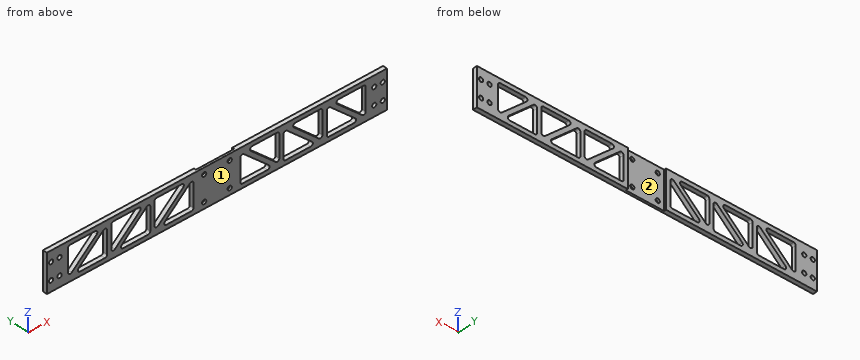
```python
from build123d import *

# Parameters (mm, degrees)
SKETCH2_W                   = 57.15
SKETCH2_H                   = 6.35
BOSS_EXTRUDE2_DEPTH         = 254
F_1_4_0_25_DIAMETER_HOLE1_D = 6.35
CUT_EXTRUDE1_REACH          = 257.681
FILLET1_R                   = 3.175
FILLET1_OF_MIRROR4_R        = 3.175
SKETCH7_W                   = 57.15
SKETCH7_H                   = 57.15
CUT_EXTRUDE2_DEPTH          = 3.175
F_1_4_0_25_DIAMETER_HOLE2_D = 6.35


with BuildPart() as part:
    # Sketch2 → Boss-Extrude2 (new, symmetric)
    with BuildSketch(Plane(origin=(0, 0, 0), x_dir=(0, 0, -1), z_dir=(1, 0, 0))):
        Rectangle(SKETCH2_W, SKETCH2_H)
    extrude(amount=BOSS_EXTRUDE2_DEPTH, both=True)

    # 1/4 (0.25) Diameter Hole1 (through all)
    with Locations(Plane(origin=(0, 3.175, 0), x_dir=(1, 0, 0), z_dir=(0, 1, 0))):
        with Locations((-247.65, -12.7), (-247.65, 12.7), (-234.95, 12.7), (-234.95, -12.7)):
            f_1_4_0_25_diameter_hole1 = Hole(F_1_4_0_25_DIAMETER_HOLE1_D / 2)

    # Mirror1: 1/4 (0.25) Diameter Hole1 across plane
    add(f_1_4_0_25_diameter_hole1.mirror(Plane(origin=(0, 0, 0), x_dir=(0, 0, 1), z_dir=(1, 0, 0))), mode=Mode.SUBTRACT)

    # Sketch6 → Cut-Extrude1 (cut, up to next)
    with BuildSketch(Plane(origin=(0, 3.175, 0), x_dir=(1, 0, 0), z_dir=(0, 1, 0)), mode=Mode.PRIVATE) as cut_extrude1_sk1:
        Polygon((-222.25, 22.225), (-222.25, -22.225), (-173.469521198, -22.225), align=None)
    cut_extrude1_tool1 = extrude(cut_extrude1_sk1.sketch, amount=-CUT_EXTRUDE1_REACH, mode=Mode.PRIVATE) & part.part
    # Sketch6 → Cut-Extrude1 (cut, up to next)
    with BuildSketch(Plane(origin=(0, 3.175, 0), x_dir=(1, 0, 0), z_dir=(0, 1, 0)), mode=Mode.PRIVATE) as cut_extrude1_sk2:
        Polygon((-212.822145469, 22.225), (-164.041666667, -22.225), (-164.041666667, 22.225), align=None)
    cut_extrude1_tool2 = extrude(cut_extrude1_sk2.sketch, amount=-CUT_EXTRUDE1_REACH, mode=Mode.PRIVATE) & part.part
    # Sketch6 → Cut-Extrude1 (cut, up to next)
    with BuildSketch(Plane(origin=(0, 3.175, 0), x_dir=(1, 0, 0), z_dir=(0, 1, 0)), mode=Mode.PRIVATE) as cut_extrude1_sk3:
        Polygon((-157.691666667, 22.225), (-157.691666667, -22.225), (-108.911187865, -22.225), align=None)
    cut_extrude1_tool3 = extrude(cut_extrude1_sk3.sketch, amount=-CUT_EXTRUDE1_REACH, mode=Mode.PRIVATE) & part.part
    # Sketch6 → Cut-Extrude1 (cut, up to next)
    with BuildSketch(Plane(origin=(0, 3.175, 0), x_dir=(1, 0, 0), z_dir=(0, 1, 0)), mode=Mode.PRIVATE) as cut_extrude1_sk4:
        Polygon((-148.263812135, 22.225), (-99.483333333, -22.225), (-99.483333333, 22.225), align=None)
    cut_extrude1_tool4 = extrude(cut_extrude1_sk4.sketch, amount=-CUT_EXTRUDE1_REACH, mode=Mode.PRIVATE) & part.part
    # Sketch6 → Cut-Extrude1 (cut, up to next)
    with BuildSketch(Plane(origin=(0, 3.175, 0), x_dir=(1, 0, 0), z_dir=(0, 1, 0)), mode=Mode.PRIVATE) as cut_extrude1_sk5:
        Polygon((-93.133333333, 22.225), (-93.133333333, -22.225), (-44.352854531, -22.225), align=None)
    cut_extrude1_tool5 = extrude(cut_extrude1_sk5.sketch, amount=-CUT_EXTRUDE1_REACH, mode=Mode.PRIVATE) & part.part
    # Sketch6 → Cut-Extrude1 (cut, up to next)
    with BuildSketch(Plane(origin=(0, 3.175, 0), x_dir=(1, 0, 0), z_dir=(0, 1, 0)), mode=Mode.PRIVATE) as cut_extrude1_sk6:
        Polygon((-83.705478802, 22.225), (-34.925, -22.225), (-34.925, 22.225), align=None)
    cut_extrude1_tool6 = extrude(cut_extrude1_sk6.sketch, amount=-CUT_EXTRUDE1_REACH, mode=Mode.PRIVATE) & part.part
    cut_extrude1_1 = cut_extrude1_tool1.solids().sort_by_distance((-205.98984, 3.175, 7.408333))[0]
    add(cut_extrude1_1, mode=Mode.SUBTRACT)
    cut_extrude1_2 = cut_extrude1_tool2.solids().sort_by_distance((-180.301826, 3.175, -7.408333))[0]
    add(cut_extrude1_2, mode=Mode.SUBTRACT)
    cut_extrude1_3 = cut_extrude1_tool3.solids().sort_by_distance((-141.431507, 3.175, 7.408333))[0]
    add(cut_extrude1_3, mode=Mode.SUBTRACT)
    cut_extrude1_4 = cut_extrude1_tool4.solids().sort_by_distance((-115.743493, 3.175, -7.408333))[0]
    add(cut_extrude1_4, mode=Mode.SUBTRACT)
    cut_extrude1_5 = cut_extrude1_tool5.solids().sort_by_distance((-76.873174, 3.175, 7.408333))[0]
    add(cut_extrude1_5, mode=Mode.SUBTRACT)
    cut_extrude1_6 = cut_extrude1_tool6.solids().sort_by_distance((-51.18516, 3.175, -7.408333))[0]
    add(cut_extrude1_6, mode=Mode.SUBTRACT)
    cut_extrude1 = cut_extrude1_1 + cut_extrude1_2 + cut_extrude1_3 + cut_extrude1_4 + cut_extrude1_5 + cut_extrude1_6  # Cut-Extrude1 as one shape, for the pattern or mirror that repeats it

    # Fillet1
    fillet1_edges = [part.edges().sort_by_distance(p)[0] for p in [
        (-93.133333333, 0, -22.225),
        (-44.352854531, 0, 22.225),
        (-93.133333333, 0, 22.225),
        (-83.705478802, 0, -22.225),
        (-34.925, 0, -22.225),
        (-34.925, 0, 22.225),
        (-222.25, 0, -22.225),
        (-173.469521198, 0, 22.225),
        (-222.25, 0, 22.225),
        (-212.822145469, 0, -22.225),
        (-164.041666667, 0, -22.225),
        (-164.041666667, 0, 22.225),
        (-157.691666667, 0, -22.225),
        (-108.911187865, 0, 22.225),
        (-157.691666667, 0, 22.225),
        (-148.263812135, 0, -22.225),
        (-99.483333333, 0, -22.225),
        (-99.483333333, 0, 22.225),
    ]]
    fillet(fillet1_edges, radius=FILLET1_R)

    # Mirror4: Cut-Extrude1 across plane
    add(cut_extrude1.mirror(Plane(origin=(0, 0, 0), x_dir=(0, 0, 1), z_dir=(1, 0, 0))), mode=Mode.SUBTRACT)

    # Fillet1 of Mirror4
    fillet1_of_mirror4_edges = [part.edges().sort_by_distance(p)[0] for p in [
        (93.133333333, 0, -22.225),
        (44.352854531, 0, 22.225),
        (93.133333333, 0, 22.225),
        (83.705478802, 0, -22.225),
        (34.925, 0, -22.225),
        (34.925, 0, 22.225),
        (222.25, 0, -22.225),
        (173.469521198, 0, 22.225),
        (222.25, 0, 22.225),
        (212.822145469, 0, -22.225),
        (164.041666667, 0, -22.225),
        (164.041666667, 0, 22.225),
        (157.691666667, 0, -22.225),
        (108.911187865, 0, 22.225),
        (157.691666667, 0, 22.225),
        (148.263812135, 0, -22.225),
        (99.483333333, 0, -22.225),
        (99.483333333, 0, 22.225),
    ]]
    fillet(fillet1_of_mirror4_edges, radius=FILLET1_OF_MIRROR4_R)

    # Sketch7 → Cut-Extrude2 (cut)
    with BuildSketch(Plane(origin=(0, 3.175, 0), x_dir=(1, 0, 0), z_dir=(0, 1, 0))):
        Rectangle(SKETCH7_W, SKETCH7_H)
    extrude(amount=-CUT_EXTRUDE2_DEPTH, mode=Mode.SUBTRACT)

    # 1/4 (0.25) Diameter Hole2 (through all)
    with Locations(Plane(origin=(0, 0, 0), x_dir=(1, 0, 0), z_dir=(0, 1, 0))):
        with Locations((19.05, -19.05), (-19.05, 19.05), (-19.05, -19.05), (19.05, 19.05)):
            Hole(F_1_4_0_25_DIAMETER_HOLE2_D / 2)


solid = part.part
```
Geometry: final body of the model. Coordinates: model frame, mm. Face numbers are marked on the shaded views. Round coordinates to 2 decimals unless told otherwise and drop trailing zeros. Use one line per item in the form item = value. Start each with the question number.
1. Draft query along X for the marked faces 1 and 2. Return one class per face: pulls with the +X half, pulls with the -X half, needs draft (parallel to the pull), parting line crosses it, or undercut.
2. Line query: probe 1 along Z at (x, y) = (247.65, 0.5) (3 decimals); probe 2 along Z at (x, y) = (-19.05, -1.1) (3 decimals); probe 3 along Z at (x, y) = (-170, -2.25) (3 decimals). Output: solid intervals per line, ascending.
3. Cut plane A-A (y = 1.25). Count the separate pieces of the cut face and the enclosed holes in it, then the cut area to 3 significant figures.
Solution:
q1.face_1 = needs draft
q1.face_2 = undercut
q2.probe_1 = -28.575 to -15.875, -9.525 to 9.525, 15.875 to 28.575
q2.probe_2 = -28.575 to -22.225, -15.875 to 15.875, 22.225 to 28.575
q2.probe_3 = -28.575 to -22.225, 16.796 to 28.575
q3.separate_pieces = 2
q3.enclosed_holes = 20
q3.area = 12,800 mm^2
